CAD build for the part. Positions are in the model's coordinates, mm. Face numbers are marked on the shaded views. A direction names the side the tool comes from. Coordinates: 2 decimals unless noted, no trailing zeros. Write each loop counter-clockwise with the first axis right and the second up, starting at its lowest first coordinate (ties: lowest second). Pieces come first, ordered by that corner, then holes. Notation, with made-up numbers: M -6,-24.75 L 8,-24.75 A20 cw 8,7.25 Z; hole C -24.5,32 d8. An arc over 180 degrees is marked long. Put each result on its own line as item: value. Start each with the question number.
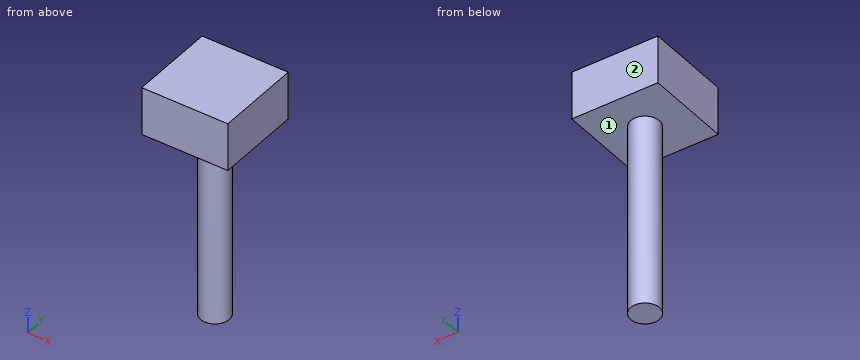
```python
from build123d import *

# Parameters (mm, degrees)
SKETCH_W     = 9
SKETCH_H     = 9
PAD_DEPTH    = 5
SKETCH001_R  = 1.5
PAD001_DEPTH = 20
SKETCH002_W  = 7
SKETCH002_H  = 7
POCKET_DEPTH = 3


with BuildPart() as part:
    # Sketch → Pad (new body)
    with BuildSketch(Plane.XY):
        Rectangle(SKETCH_W, SKETCH_H)
    extrude(amount=PAD_DEPTH)

    # Sketch001 (on Face5 of Pad) → Pad001 (join)
    with BuildSketch(Plane(origin=(0, 0, 0), x_dir=(1, 0, 0), z_dir=(0, 0, -1))):
        Circle(SKETCH001_R)
    extrude(amount=PAD001_DEPTH)

    # Sketch002 → Pocket (cut)
    with BuildSketch(Plane.XY.offset(4)):
        Rectangle(SKETCH002_W, SKETCH002_H)
    extrude(amount=-POCKET_DEPTH, mode=Mode.SUBTRACT)


solid = part.part
```
(1) Drill centre lines: line 1 (Z direction, x = 1.5, y = -1); line 2 (X direction, y = -2.5, z = 2.75); line 3 (Z direction, x = 4, y = 4.25). Where is each one in solid material? Low to high. Write a range as [from, to].
(2) Slice it at B-B, the plane z = 2.75. Write the cut outline in (x, y), then the cut area to 3 significant figures.
(3) Which spindle directions (+Z, -Z, +X, -X, +Y, -Y) get a long thin tool onto all of the face, cutting with end or side? Do the marked faces 1 and 2. Say none if no direction does.
(4) Slice it at A-A, the plane y = -2. Write the cut outline in (x, z), then the cut area to 3 significant figures.
(5) Slice it at C-C, the plane x = 0. Write the cut outline in (y, z), then the cut area to 3 significant figures.
(6) Drop a flat-ended pin along its axis: pin 1 (1.5 mm diameter, centred on y = 1.5, z = -8.5, fed in from -X). Give the stop position or say it passes through.
Result set:
1. line 1: z = [0, 1], [4, 5]
1. line 2: x = [-4.5, -3.5], [3.5, 4.5]
1. line 3: z = [0, 5]
2. outline: M -4.5,-4.5 L 4.5,-4.5 L 4.5,4.5 L -4.5,4.5 Z; hole M -3.5,-3.5 L 3.5,-3.5 L 3.5,3.5 L -3.5,3.5 Z
2. area: 32.0 mm^2
3. face 1: -Z
3. face 2: +Z, -Z, +X, -X, +Y
4. outline: M -4.5,0 L 4.5,0 L 4.5,5 L -4.5,5 Z; hole M -3.5,1 L 3.5,1 L 3.5,4 L -3.5,4 Z
4. area: 24.0 mm^2
5. outline: M -4.5,0 L -1.5,0 L -1.5,-20 L 1.5,-20 L 1.5,0 L 4.5,0 L 4.5,5 L -4.5,5 Z; hole M -3.5,1 L 3.5,1 L 3.5,4 L -3.5,4 Z
5. area: 84.0 mm^2
6. pin 1: stops at x = -1.3
